```python
from build123d import *

# Parameters (mm, degrees)
CROQUIS1_W                   = 50
CROQUIS1_H                   = 30
SALIENTE_EXTRUIR1_DEPTH      = 3
SALIENTE_EXTRUIR2_DEPTH      = 15
SALIENTE_EXTRUIR2_DEPTH_BACK = 15
CORTAR_EXTRUIR1_DEPTH        = 60.741108125
CROQUIS4_R                   = 2.5
SALIENTE_EXTRUIR3_DEPTH      = 10


with BuildPart() as part:
    # Croquis1 → Saliente-Extruir1 (new body)
    with BuildSketch(Plane.XY):
        with Locations((25, 15)):
            Rectangle(CROQUIS1_W, CROQUIS1_H)
    extrude(amount=SALIENTE_EXTRUIR1_DEPTH)

    # Croquis2 → Saliente-Extruir2 (add, two sides: drawn at the far end of the back side and taken through both)
    with BuildSketch(Plane(origin=(0, 15, 0), x_dir=(1, 0, 0), z_dir=(0, 1, 0)).offset(-SALIENTE_EXTRUIR2_DEPTH_BACK)):
        with BuildLine():
            Line((15, -3), (35, -3))
            ThreePointArc((35, -3), (25, -13), (15, -3))
        make_face()
    extrude(amount=SALIENTE_EXTRUIR2_DEPTH + SALIENTE_EXTRUIR2_DEPTH_BACK)

    # Croquis3 → Cortar-Extruir1 (cut, through all)
    with BuildSketch(Plane(origin=(0, 30, 0), x_dir=(1, 0, 0), z_dir=(0, 1, 0))):
        with BuildLine():
            ThreePointArc((17.281029865, -9.357475919), (18.433447729, -9.235618719), (19.413280597, -8.616875104))
            ThreePointArc((19.413280597, -8.616875104), (20.164937796, -8.08539476), (21.05409871, -7.846956572))
            ThreePointArc((21.05409871, -7.846956572), (21.364087604, -8.083627253), (21.688234212, -8.300503029))
            ThreePointArc((21.688234212, -8.300503029), (21.719260259, -9.423145978), (21.277056507, -10.455495555))
            ThreePointArc((21.277056507, -10.455495555), (21.160716532, -11.401170735), (21.390501043, -12.325852094))
            ThreePointArc((21.390501043, -12.325852094), (19.144543803, -11.106394558), (17.281029865, -9.357475919))
        make_face()
        with BuildLine():
            ThreePointArc((17.605845109, -6.843331325), (18.570395316, -6.268063818), (19.205167685, -5.34158994))
            ThreePointArc((19.205167685, -5.34158994), (19.070403954, -4.975605156), (18.958729207, -4.601927653))
            ThreePointArc((18.958729207, -4.601927653), (18.099232466, -4.272192527), (17.17873271, -4.260356141))
            ThreePointArc((17.17873271, -4.260356141), (16.022342896, -4.184998931), (15.018391395, -3.606209252))
            ThreePointArc((15.018391395, -3.606209252), (15.498017257, -6.116460163), (16.598255677, -8.423162576))
            ThreePointArc((16.598255677, -8.423162576), (16.955870168, -7.540015696), (17.605845109, -6.843331325))
        make_face()
        with BuildLine():
            ThreePointArc((22.492052569, -12.680402868), (23.35275234, -11.904444098), (23.781765411, -10.827938688))
            ThreePointArc((23.781765411, -10.827938688), (24.07747255, -9.956149042), (24.65666839, -9.240612823))
            ThreePointArc((24.65666839, -9.240612823), (25.046566209, -9.249876526), (25.436282706, -9.234804119))
            ThreePointArc((25.436282706, -9.234804119), (26.121256275, -10.12480469), (26.370305781, -11.219913886))
            ThreePointArc((26.370305781, -11.219913886), (26.832038689, -12.053364099), (27.561452328, -12.666383086))
            ThreePointArc((27.561452328, -12.666383086), (25.027655598, -12.999961758), (22.492052569, -12.680402868))
        make_face()
        with BuildLine():
            ThreePointArc((28.661025949, -12.305744946), (28.90124957, -11.172074481), (28.615574431, -10.048995755))
            ThreePointArc((28.615574431, -10.048995755), (28.342381435, -9.16989082), (28.390379076, -8.250567086))
            ThreePointArc((28.390379076, -8.250567086), (28.711258105, -8.028885391), (29.017686036, -7.787621948))
            ThreePointArc((29.017686036, -7.787621948), (30.094970504, -8.105030174), (30.940144821, -8.844604497))
            ThreePointArc((30.940144821, -8.844604497), (31.803584335, -9.24748009), (32.754015885, -9.314684288))
            ThreePointArc((32.754015885, -9.314684288), (30.900203893, -11.073883453), (28.661025949, -12.305744946))
        make_face()
        with BuildLine():
            ThreePointArc((33.43161185, -8.376608746), (32.959602062, -7.318250172), (32.068356907, -6.57757603))
            ThreePointArc((32.068356907, -6.57757603), (31.330614215, -6.026944012), (30.829080189, -5.254983182))
            ThreePointArc((30.829080189, -5.254983182), (30.958375546, -4.887030963), (31.064469856, -4.511730919))
            ThreePointArc((31.064469856, -4.511730919), (32.122579172, -4.135307644), (33.241050438, -4.236854841))
            ThreePointArc((33.241050438, -4.236854841), (34.17639201, -4.05527103), (34.984808923, -3.55099072))
            ThreePointArc((34.984808923, -3.55099072), (34.519074843, -6.06385609), (33.43161185, -8.376608746))
        make_face()
    extrude(amount=-CORTAR_EXTRUIR1_DEPTH, mode=Mode.SUBTRACT)

    # Croquis4 → Saliente-Extruir3 (add)
    with BuildSketch(Plane(origin=(0, 30, 0), x_dir=(1, 0, 0), z_dir=(0, 1, 0))):
        with Locations(Location((25, -3, 0), (0, 0, 90))):
            Circle(CROQUIS4_R)
    saliente_extruir3 = extrude(amount=SALIENTE_EXTRUIR3_DEPTH)

    # Simetría2: Saliente-Extruir3 across plane
    add(saliente_extruir3.mirror(Plane.ZX.offset(15)))


solid = part.part
```
Read the model definition and answer for the solid it produces. Units are mm, in the model's axes. A direction names the side the tool comes from. Give positions to 0.01 mm unless a question says otherwise; leave off trailing zeros. Write each loop counter-clockwise with the first axis right and the second up, starting at its lowest first coordinate (ties: lowest second). Pieces come first, ordered by that corner, then holes. Notation, with made-up numbers: (38.25, 60) -> (93.25, 60) arc R6 ccw to (93.25, 68) -> close; hole circle Ø6 at (-20.75, -24.5). An arc over 180 degrees is marked (long way). Answer in a Markdown table with one row per item.
1) Straight lines are drawn through the part: line 1 (Z direction, x = 33.5, y = 7); line 2 (Z direction, x = 37, y = 9.5); line 3 (Y direction, x = 34, z = 3.25). For each, find the intervals that lie inside material, in ascending order. Write a range as [from, to].
Results list:
| item | result |
|---|---|
| line 1 | [0, 4.22] |
| line 2 | [0, 3] |
| line 3 | [0, 30] |
2) A tool of negligible diameter and unlimited length cuts with its end or side. For faces 1 (the cylindrical face through (32.97, 15.21, 7.33)), 2 (the flat face through (7, 15, 3)), 3 (the cylindrical face through (21.72, 15.21, 9.41)), from which of +Z, -Z, +X, -X, +Y, -Y can it reach the whole face along a straight path? Write none if from no direction.
Results list:
| item | result |
|---|---|
| face 1 | +X, +Y, -Y |
| face 2 | +Z, -X, +Y, -Y |
| face 3 | +Y, -Y |
3) Section A-A on y = -5.5 is taken. Give the vertices of the cut face in (x, z), plus the area to 3 significant figures.
Results list:
| item | result |
|---|---|
| outline | circle Ø5 at (25, 3) |
| area | 19.6 mm^2 |
4) Section C-C on x = 20 is taken. Give the vertices of the cut face in (y, z).
Results list:
| item | result |
|---|---|
| outline | (0, 0) -> (30, 0) -> (30, 8.17) -> (0, 8.17) -> close |
5) Section B-B on x = 5.5 is taken. Give the vertices of the cut face in (y, z).
Results list:
| item | result |
|---|---|
| outline | (0, 0) -> (30, 0) -> (30, 3) -> (0, 3) -> close |
6) Each of these flat-tipped pins is pushed along its axis until it touches: pin 1 Ø5 at (y, z) = (18.5, 7) entering from -X; pin 2 Ø4.5 at (x, y) = (11, 9) entering from +Z; pin 3 Ø6 at (y, z) = (-4.5, 10) entering from -X; pin 4 Ø6 at (x, z) = (35, 8.5) entering from -Y. Where does it stop, or does it pass through?
Results list:
| item | result |
|---|---|
| pin 1 | x = 16.6 |
| pin 2 | z = 3 |
| pin 3 | through |
| pin 4 | y = 0 |
7) Determine the mould class of faces 4 (the cylindrical face through (32.107, 15.21, 4.137)), 5 (the cylindrical face through (20.153, 15.21, 8.091)), 6 (the cylindrical face through (22.52, 34.93, 3.33)) for opening direction Z: released by +Z, released by -Z, zero draft, split by the parting line, or undercut.
Results list:
| item | result |
|---|---|
| face 4 | undercut |
| face 5 | released by +Z |
| face 6 | split by the parting line |
